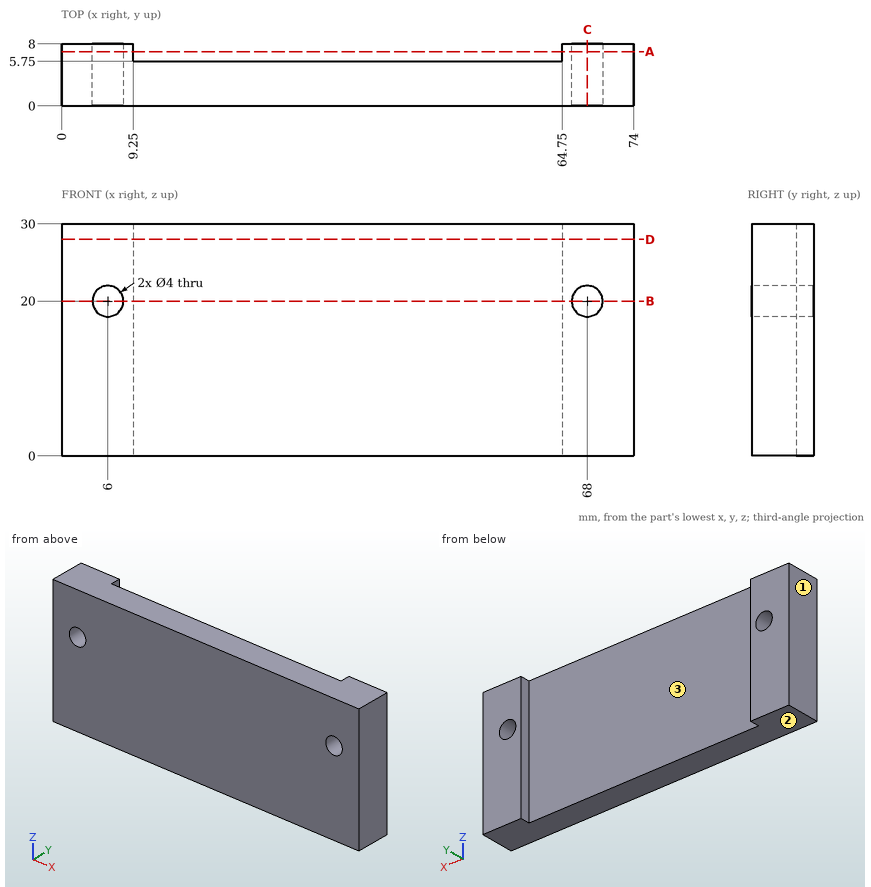
The figure shows three views and two pictorial views of one solid part (mm, origin at its lowest corner). Answer the questions. Give positions to 0.01 mm unless a question says otherwise; leave off trailing zeros. Loops run counter-clockwise (first coordinate to the right, second up) from the corner with the lowest first, then second, coordinate; pieces in that order, holes last. Notation, with made-up numbers: (77, 18.5) -> (92, 18.5) arc R21 ccw to (92, 55.5) -> close; hole circle Ø2 at (-26.75, 37.25). An arc over 180 degrees is marked (long way). Put each result on its own line as item: value. Start each with the question number.
Item 1: This flat-tipped pin is pushed along its axis until it touches: P1, Ø10, axis at x = 27, z = 7.5, coming from the +Y side. Where does it stop, or does it pass through?
Item 2: The mould has two halves that part along X. Classify the marked faces 1, 2 and 3: released by +X, released by -X, zero draft, split by the parting line, or undercut.
Item 3: The part is cut by section C-C (x = 68). Give the vertices of the cut face in (y, z).
Item 4: The part is cut by section A-A (y = 7). Give the vertices of the cut face in (x, z).
Item 5: The part is cut by section D-D (z = 28). Give the vertices of the cut face in (x, y).
Item 6: The part is cut by section B-B (z = 20). Give the vertices of the cut face in (x, y).
Item 7: Find the intervals of material crossed by L1, parallel to X at y = 3.5, z = 20; L2, parallel to X at y = 6, z = 20; L3, parallel to Z at x = 6, y = 2.5, in increasing order. Write a range as [from, to].
Answers below:
1. P1: y = 5.75
2. face 1: released by -X
2. face 2: zero draft
2. face 3: undercut
3. outline: (0, 0) -> (8, 0) -> (8, 18) -> (0, 18) -> close; (0, 22) -> (8, 22) -> (8, 30) -> (0, 30) -> close
4. outline: (0, 0) -> (9.25, 0) -> (9.25, 30) -> (0, 30) -> close; (64.75, 0) -> (74, 0) -> (74, 30) -> (64.75, 30) -> close; hole circle Ø4 at (6, 20); hole circle Ø4 at (68, 20)
5. outline: (0, 0) -> (74, 0) -> (74, 8) -> (64.75, 8) -> (64.75, 5.75) -> (9.25, 5.75) -> (9.25, 8) -> (0, 8) -> close
6. outline: (0, 0) -> (4, 0) -> (4, 8) -> (0, 8) -> close; (8, 0) -> (66, 0) -> (66, 8) -> (64.75, 8) -> (64.75, 5.75) -> (9.25, 5.75) -> (9.25, 8) -> (8, 8) -> close; (70, 0) -> (74, 0) -> (74, 8) -> (70, 8) -> close
7. L1: [0, 4], [8, 66], [70, 74]
7. L2: [0, 4], [8, 9.25], [64.75, 66], [70, 74]
7. L3: [0, 18], [22, 30]
